Check sheet for the modelled part. Datum: model origin and axes. Units: mm. A direction names the side the tool comes from. Round coordinates to 2 decimals unless told otherwise and drop trailing zeros. Write each loop counter-clockwise with the first axis right and the second up, starting at its lowest first coordinate (ties: lowest second). Pieces come first, ordered by that corner, then holes.
Item 1: Section check C-C, the plane x = 6.5. Record the cut outline in (y, z), plus the area to 3 significant figures.
Item 2: Set-up check for faces 4 (the flat face through (-4, 18, 51)), 5 (the flat face through (6, 0, 42)): record each of +Z, -Z, +X, -X, +Y, -Y from which the full face is reachable in a straight line by a thin tool's end or side.
Item 3: Release check for a two-part mould opening along Y. For faces 1 (the cylindrical face through (-1.972, 23.675, 31.325)), 2 (the flat face through (-2, 42.3, 57)), 3 (the flat face through (0, 21, 51)) record: pulls with the +Y half, pulls with the -Y half, needs draft (parallel to the pull), parting line crosses it, or undercut.
Item 4: Section check D-D, the plane z = 9. Record the cut outline in (x, y).
Item 5: Section check B-B, the plane y = 24.5. Record the cut outline in (x, z).
Item 6: Material ranges on line 1 along Y through (x, z) = (5.75, 33); line 2 along X through (y, z) = (5, 59); line 3 along Z through (x, y) = (-0.25, 9), recorded low to high.
Item 7: Depth check by flat-ended pin: pin 1 (4 mm diameter, centred on x = 3.5, y = 3.5, fed in from -Z). Enter the tip coordinate at first touch or a pass-through.
Item 8: Section check A-A, the plane z = 33.5. Record the cut outline in (x, y).
from build123d import *

# Parameters (mm, degrees)
EXTRUDE_1_DEPTH     = 85
SKETCH_2_R          = 3
CUT_EXTRUDE_1_DEPTH = 96.698955062
CHAMFER_1_SIZE      = 35
CHAMFER_2_SIZE      = 5


with BuildPart() as part:
    # Эскиз1 → Вытянуть1 (new body)
    with BuildSketch(Plane.XY):
        Polygon((0, 0), (12, 0), (12, -5), (-4, -5), (-4, 42.3), (0, 42.3), align=None)
    extrude(amount=EXTRUDE_1_DEPTH)

    # Эскиз2 → Вырез-Вытянуть1 (cut, through all)
    with BuildSketch(Plane(origin=(0, 0, 0), x_dir=(0, 0, -1), z_dir=(1, 0, 0))):
        with Locations((-34.186530765, 22.773427237)):
            Circle(SKETCH_2_R)
    extrude(amount=-CUT_EXTRUDE_1_DEPTH, mode=Mode.SUBTRACT)

    # Фаска1
    chamfer_1_edges = [part.edges().sort_by_distance(p)[0] for p in [
        (-2, 42.3, 0),
    ]]
    chamfer(chamfer_1_edges, length=CHAMFER_1_SIZE)

    # Фаска2
    chamfer_2_edges = [part.edges().sort_by_distance(p)[0] for p in [
        (-2, 42.3, 85),
    ]]
    chamfer(chamfer_2_edges, length=CHAMFER_2_SIZE)


solid = part.part
Values found:
1. outline: (-5, 0) - (0, 0) - (0, 85) - (-5, 85) - close
1. area: 425 mm2
2. face 4: +Z, -Z, -X, +Y, -Y
2. face 5: +Z, -Z, +X, +Y
3. face 1: undercut
3. face 2: pulls with the +Y half
3. face 3: needs draft
4. outline: (-4, -5) - (12, -5) - (12, 0) - (0, 0) - (0, 16.3) - (-4, 16.3) - close
5. outline: (-4, 17.2) - (0, 17.2) - (0, 31.73) - (-4, 31.73) - close; (-4, 36.64) - (0, 36.64) - (0, 85) - (-4, 85) - close
6. line 1: y = -5 to 0
6. line 2: x = -4 to 0
6. line 3: z = 1.7 to 85
7. pin 1: passes through
8. outline: (-4, -5) - (12, -5) - (12, 0) - (0, 0) - (0, 19.85) - (-4, 19.85) - close; (-4, 25.69) - (0, 25.69) - (0, 40.8) - (-4, 40.8) - close
